Part model, mm, in its own coordinate system. Give positions to 0.01 mm unless a question says otherwise; leave off trailing zeros. Write each loop counter-clockwise with the first axis right and the second up, starting at its lowest first coordinate (ties: lowest second). Pieces come first, ordered by that corner, then holes. Notation, with made-up numbers: (24.25, -0.75) - (60.25, -0.75) arc R17 ccw to (60.25, 20.25) - close; hole circle Ø3 at (-11, -2). An arc over 180 degrees is marked (long way). Answer in a Markdown table with one row per item. Add a question column.
1. Band-saw the part on A-A on y = 163. Write the cut outline in (x, z).
2. Band-saw the part on C-C on z = 597. Write the cut outline in (x, y).
3. Band-saw the part on B-B on x = 810. Write the cut outline in (y, z), plus the area to 3 significant figures.
4. Probe line 1 along Y through (x, z) = (-702.5, -235.5); line 2 along Z through (x, y) = (365, 45); line 3 along Z through (x, y) = (-186.5, 147.5). List the from-to ranges inside material, lowest first.
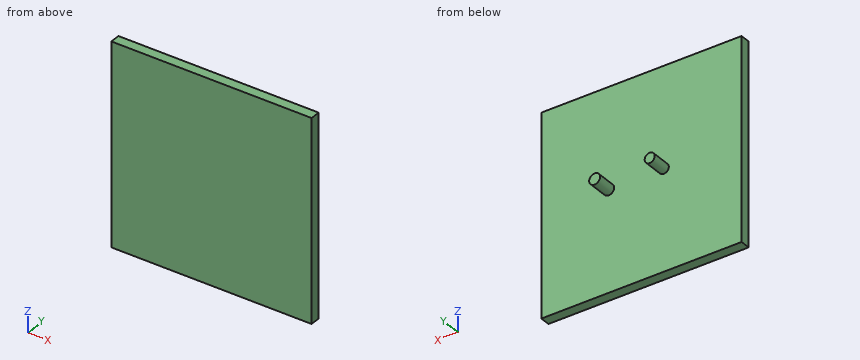
```python
from build123d import *

# Parameters (mm, degrees)
F0_W     = 2000
F0_H     = 2000
F1_DEPTH = 100
F2_R     = 50
F2_R_2   = 54.251407
F3_DEPTH = 300


with BuildPart() as f1:
    # F0 (on Front) → F1 (new body)
    with BuildSketch(Plane.XZ):
        with Locations((-8.939937, 483.27489)):
            Rectangle(F0_W, F0_H)
    extrude(amount=F1_DEPTH)

    # F2 (on face) → F3 (join)
    with BuildSketch(Plane.XZ.offset(100)):
        with Locations((-232.198777, 483.27489)):
            Circle(F2_R)
        with Locations((317.801223, 483.27489)):
            Circle(F2_R_2)
    extrude(amount=-F3_DEPTH)


solid = f1.part
```
Values:
| question | item | result |
|---|---|---|
| 1 | outline | circle Ø100 at (-232.2, 483.27); circle Ø108.5 at (317.8, 483.27) |
| 2 | outline | (-1008.94, -100) - (991.06, -100) - (991.06, 0) - (-1008.94, 0) - close |
| 3 | outline | (-100, -516.73) - (0, -516.73) - (0, 1483.27) - (-100, 1483.27) - close |
| 3 | area | 200,000 mm² |
| 4 | line 1 | y = -100 to 0 |
| 4 | line 2 | z = 456.53 to 510.02 |
| 4 | line 3 | z = 462.99 to 503.56 |
